The figure shows three views and two pictorial views of one solid part (mm, origin at its lowest corner). Answer the questions. A direction names the side the tool comes from. Coordinates: 2 decimals unless noted, no trailing zeros. Write each loop counter-clockwise with the first axis right and the second up, starting at its lowest first coordinate (ties: lowest second). Pieces come first, ordered by that corner, then holes. Notation, with made-up numbers: M 87,-6 L 132,-6 A18 cw 132,10 Z; hole C -26,77 d4. An arc over 180 degrees is marked long. Answer as CSV lines item,"result".
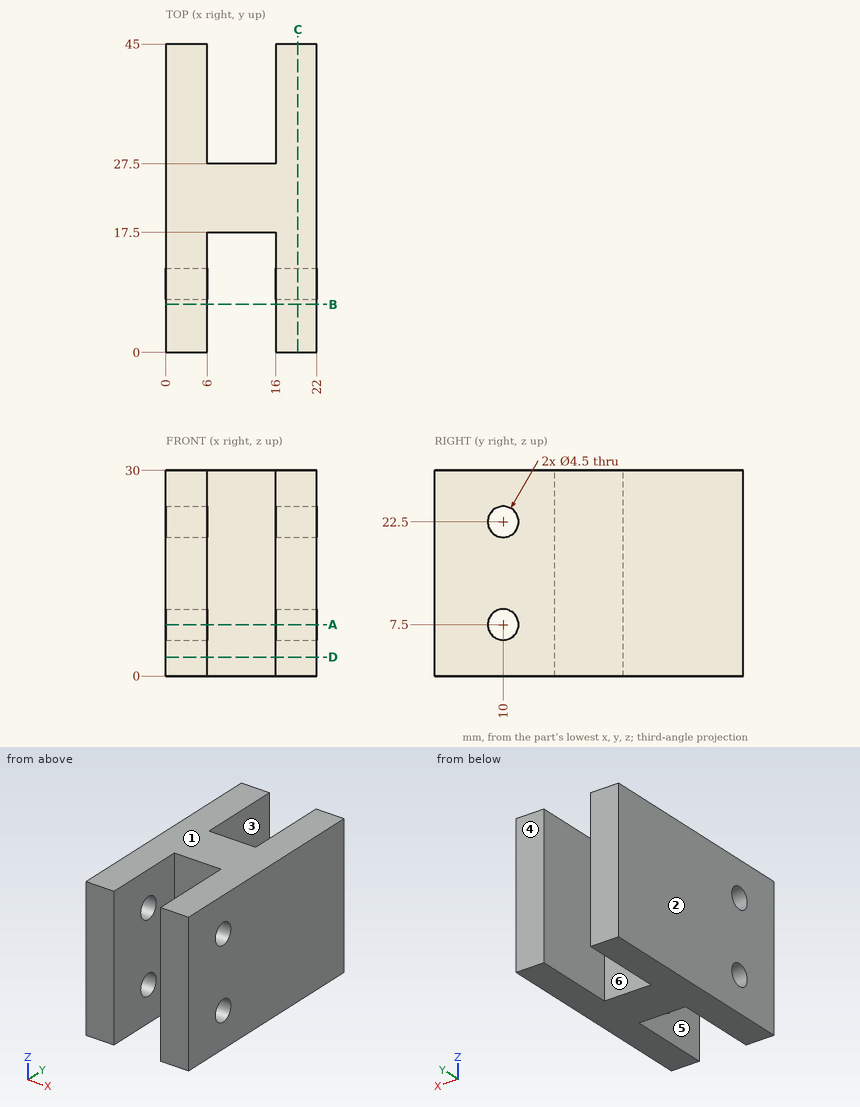
Q1. Find section D-D (z = 2.75). Give the vertices of the cut face in (x, y), and give its area (3 significant figures).
Output:
outline,"M 0,0 L 6,0 L 6,17.5 L 16,17.5 L 16,0 L 22,0 L 22,45 L 16,45 L 16,27.5 L 6,27.5 L 6,45 L 0,45 Z"
area,"640 mm2"
Q2. Straight lines are drawn through the part: line 1 (Z direction, x = 20.5, y = 10); line 2 (X direction, y = 33, z = 19.25); line 3 (Y direction, x = 12.25, z = 25.5). For each, find the intervals that lie inside material, in ascending order.
Output:
line 1,"0 to 5.25, 9.75 to 20.25, 24.75 to 30"
line 2,"0 to 6, 16 to 22"
line 3,"17.5 to 27.5"
Q3. Flat-ended cylindrical pins translate along their axes: pin 1 Ø6 at (x, z) = (8.5, 5) entering from +Y; pin 2 Ø4 at (y, z) = (10, 7.5) entering from -X; pin 3 Ø5 at (x, z) = (9.5, 14.5) entering from -Y. Find the tip coordinate at first contact, or state that the pin passes through.
Output:
pin 1,"y = 45"
pin 2,"through"
pin 3,"y = 17.5"
Q4. Find section A-A (z = 7.5). Give the vertices of the cut face in (x, y).
Output:
outline,"M 0,0 L 6,0 L 6,7.75 L 0,7.75 Z; M 0,12.25 L 6,12.25 L 6,17.5 L 16,17.5 L 16,12.25 L 22,12.25 L 22,45 L 16,45 L 16,27.5 L 6,27.5 L 6,45 L 0,45 Z; M 16,0 L 22,0 L 22,7.75 L 16,7.75 Z"
Q5. Find section C-C (x = 19.25). Give the vertices of the cut face in (y, z), and give its area (3 significant figures).
Output:
outline,"M 0,0 L 45,0 L 45,30 L 0,30 Z; hole C 10,7.5 d4.5; hole C 10,22.5 d4.5"
area,"1,320 mm2"
Q6. The mould has two halves that part along X. Classify the marked faces 1, 2 and 3: pulls with the +X half, pulls with the -X half, needs draft (parallel to the pull), parting line crosses it, or undercut.
Output:
face 1,"needs draft"
face 2,"pulls with the -X half"
face 3,"undercut"
Q7. Find section B-B (y = 7). Give the vertices of the cut face in (x, z).
Output:
outline,"M 0,0 L 6,0 L 6,30 L 0,30 Z; M 16,0 L 22,0 L 22,30 L 16,30 Z"
Q8. For the marked faces 4, 5 and 6, determine the directions among +Z, -Z, +X, -X, +Y, -Y from which every point of the face is accessible in a straight line to the end or side of a thin tool.
Output:
face 4,"+Z, -Z, +X, -X, +Y"
face 5,"+Z, -Z, -Y"
face 6,"+Z, -Z, +Y"
